from build123d import *

# Parameters (mm, degrees)
BOSS_EXTRUDE1_DEPTH     = 19.05
SKETCH2_W               = 42.164
SKETCH2_H               = 27.686
BOSS_EXTRUDE2_DEPTH     = 2.54
SKETCH3_W               = 7.0612
SKETCH3_H               = 14.986
BOSS_EXTRUDE3_DEPTH     = 6.35
CUT_EXTRUDE1_DEPTH      = 50.127067096
CUT_EXTRUDE1_DEPTH_BACK = 50.127067096
SKETCH4_R               = 1.75
FILLET2_R               = 1.27
CUT_EXTRUDE2_DEPTH      = 52.65763053
CUT_EXTRUDE2_DEPTH_BACK = 52.65763053
SKETCH5_R               = 4.7625
SKETCH6_W               = 25.4
SKETCH6_H               = 4.7625
BOSS_EXTRUDE4_DEPTH     = 9.525
FILLET3_R               = 3.175
FILLET4_R               = 1.27
FILLET6_R               = 1.27
CUT_EXTRUDE3_DEPTH      = 58.486687197
CUT_EXTRUDE3_DEPTH_BACK = 58.486687197
SKETCH8_R               = 2.3
SKETCH9_W               = 2.54
SKETCH9_H               = 10.16
CUT_EXTRUDE4_DEPTH      = 14.5288
CUT_EXTRUDE5_DEPTH      = 51.648644651
CUT_EXTRUDE5_DEPTH_BACK = 51.648644651
SKETCH10_R              = 1.7499965


with BuildPart() as part:
    # Sketch1 → Boss-Extrude1 (new body)
    with BuildSketch(Plane.XY):
        Polygon((-2.54, 25.146), (39.624, 25.146), (39.624, 22.606), (37.084, 22.606), (0, 22.606), (0, 0), (37.084, 0), (39.624, 0), (39.624, -2.54), (-2.54, -2.54), align=None)
    extrude(amount=BOSS_EXTRUDE1_DEPTH)

    # Sketch2 → Boss-Extrude2 (add)
    with BuildSketch(Plane.XY.offset(19.05)):
        with Locations((18.542, 11.303)):
            Rectangle(SKETCH2_W, SKETCH2_H)
    extrude(amount=BOSS_EXTRUDE2_DEPTH)

    # Sketch3 → Boss-Extrude3 (add)
    with BuildSketch(Plane.ZY.offset(2.54)):
        with Locations((18.0594, 11.303)):
            Rectangle(SKETCH3_W, SKETCH3_H)
    extrude(amount=BOSS_EXTRUDE3_DEPTH)

    # Sketch4 → Cut-Extrude1 (cut, two sides: drawn at the far end of the back side and taken through both)
    with BuildSketch(Plane(origin=(0, 0, 14.5288), x_dir=(-1, 0, 0), z_dir=(0, 0, -1)).offset(-CUT_EXTRUDE1_DEPTH_BACK)):
        with Locations(Location((4.7625, 11.303, 0), (0, 0, 90))):
            Circle(SKETCH4_R)
    extrude(amount=CUT_EXTRUDE1_DEPTH + CUT_EXTRUDE1_DEPTH_BACK, mode=Mode.SUBTRACT)

    # Fillet2
    fillet2_edges = [part.edges().sort_by_distance(p)[0] for p in [
        (-2.54, 18.796, 18.0594),
        (-2.54, 3.81, 18.0594),
        (-8.89, 18.796, 18.0594),
        (-8.89, 3.81, 18.0594),
    ]]
    fillet(fillet2_edges, radius=FILLET2_R)

    # Sketch5 → Cut-Extrude2 (cut, two sides: drawn at the far end of the back side and taken through both)
    with BuildSketch(Plane.XY.offset(21.59).offset(-CUT_EXTRUDE2_DEPTH_BACK)):
        with Locations((10.16, 11.303)):
            Circle(SKETCH5_R)
        with BuildLine():
            Line((25.4, 16.0655), (10.16, 16.0655))
            ThreePointArc((10.16, 16.0655), (13.527596045, 14.670596045), (14.9225, 11.303))
            ThreePointArc((14.9225, 11.303), (13.527596045, 7.935403955), (10.16, 6.5405))
            Line((10.16, 6.5405), (25.4, 6.5405))
            ThreePointArc((25.4, 6.5405), (20.6375, 11.303), (25.4, 16.0655))
        make_face()
        with Locations((25.4, 11.303)):
            Circle(SKETCH5_R)
    extrude(amount=CUT_EXTRUDE2_DEPTH + CUT_EXTRUDE2_DEPTH_BACK, mode=Mode.SUBTRACT)

    # Sketch6 → Boss-Extrude4 (add)
    with BuildSketch(Plane.XY.offset(21.59)):
        with Locations((26.924, 22.76475)):
            Rectangle(SKETCH6_W, SKETCH6_H)
    extrude(amount=BOSS_EXTRUDE4_DEPTH)

    # Fillet3
    fillet3_edges = [part.edges().sort_by_distance(p)[0] for p in [
        (14.224, 22.76475, 21.59),
        (14.224, 22.76475, 31.115),
        (39.624, 22.76475, 31.115),
    ]]
    fillet(fillet3_edges, radius=FILLET3_R)

    # Fillet4
    fillet4_edges = [part.edges().sort_by_distance(p)[0] for p in [
        (25.3365, 20.3835, 21.59),
    ]]
    fillet(fillet4_edges, radius=FILLET4_R)

    # Fillet6
    fillet6_edges = [part.edges().sort_by_distance(p)[0] for p in [
        (0, 0, 9.525),
        (0, 22.606, 9.525),
    ]]
    fillet(fillet6_edges, radius=FILLET6_R)

    # Sketch8 → Cut-Extrude3 (cut, two sides: drawn at the far end of the back side and taken through both)
    with BuildSketch(Plane(origin=(0, 25.146, 0), x_dir=(1, 0, 0), z_dir=(0, 1, 0)).offset(-CUT_EXTRUDE3_DEPTH_BACK)):
        with Locations(Location((20.574, -26.3525, 0), (0, 0, 270))):
            Circle(SKETCH8_R)
        with Locations(Location((33.274, -26.3525, 0), (0, 0, 270))):
            Circle(SKETCH8_R)
    extrude(amount=CUT_EXTRUDE3_DEPTH + CUT_EXTRUDE3_DEPTH_BACK, mode=Mode.SUBTRACT)

    # Sketch9 → Cut-Extrude4 (cut)
    with BuildSketch(Plane(origin=(0, 0, 0), x_dir=(-1, 0, 0), z_dir=(0, 0, -1))):
        with Locations((1.27, 11.303)):
            Rectangle(SKETCH9_W, SKETCH9_H)
    extrude(amount=-CUT_EXTRUDE4_DEPTH, mode=Mode.SUBTRACT)

    # Sketch10 → Cut-Extrude5 (cut, two sides: drawn at the far end of the back side and taken through both)
    with BuildSketch(Plane(origin=(0, 0, 19.05), x_dir=(-1, 0, 0), z_dir=(0, 0, -1)).offset(-CUT_EXTRUDE5_DEPTH_BACK)):
        with Locations(Location((-34.344, 1.95, 0), (0, 0, 180))):
            Circle(SKETCH10_R)
    extrude(amount=CUT_EXTRUDE5_DEPTH + CUT_EXTRUDE5_DEPTH_BACK, mode=Mode.SUBTRACT)


solid = part.part
Model file for the job. Use its own axes, mm. A direction names the side the tool comes from. Give positions to 0.01 mm unless a question says otherwise; leave off trailing zeros. Loops run counter-clockwise (first coordinate to the right, second up) from the corner with the lowest first, then second, coordinate; pieces in that order, holes last. Notation, with made-up numbers: (-35, -33) -> (-22, -33) arc R24 ccw to (-22, -9) -> close; hole circle Ø6 at (-5.75, 31). An arc over 180 degrees is marked (long way). Use a Markdown table: item, result. Add a question column.
(1) Tool access for faces 1 (the flat face through (18, 6.54, 20)), 2 (the flat face through (-1, 6.223, 7)), 3 (the cylindrical face through (0.36, 22.22, 9.66)): list every direction of +Z, -Z, +X, -X, +Y, -Y with a clear straight run to the whole face (end or side of a thin tool).
(2) Wall check: line 1 along Y through (x, z) = (17.5, 16); line 2 along Z through (x, y) = (10, 24.25); line 3 along Z through (x, y) = (33.5, 17.75). Give the ranges that are in metal, low to high.
(3) Slice it at A-A on y = 1.95. List the corners of the cut face in (x, z).
(4) Mould opens along X. For faces 4 (the flat face through (18, 16.066, 20)), 5 (the flat face through (-2.54, 21, 8)), 6 (the flat face through (27, 23, 31.115)) say: +X half, -X half, draft (parallel to the pull), parting line (faces both ways), or undercut.
(5) Drop flat-ended pins along their axis: pin 1 Ø3 at (x, y) = (14.5, 6.5) entering from +Z; pin 2 Ø2.5 at (x, z) = (25.5, 28) entering from -Y; pin 3 Ø11.5 at (x, y) = (27.5, 14) entering from -Z. Give the stop position or say it passes through.
(6) Slice it at D-D on x = -2. List the corners of the cut face in (y, z).
(7) Slice it at B-B on x = 15. List the corners of the cut face in (y, z), and give its area (3 significant figures).
(8) Slice it at C-C on z = 20. Give the number of separate pieces and of enclosed holes in the cut face, and give its area (3 significant figures).
Filled sheet:
| question | item | result |
|---|---|---|
| 1 | face 1 | +Z, -Z |
| 1 | face 2 | -Z, +X, -X |
| 1 | face 3 | -Z, +X |
| 2 | line 1 | -2.54 to 0, 22.61 to 25.15 |
| 2 | line 2 | 0 to 21.59 |
| 2 | line 3 | 19.05 to 21.59 |
| 3 | outline | (-2.54, 0) -> (0, 0) -> (0, 19.05) -> (32.59, 19.05) -> (32.59, 21.59) -> (-2.54, 21.59) -> close; (36.09, 19.05) -> (39.62, 19.05) -> (39.62, 21.59) -> (36.09, 21.59) -> close |
| 4 | face 4 | undercut |
| 4 | face 5 | -X half |
| 4 | face 6 | draft |
| 5 | pin 1 | z = 21.59 |
| 5 | pin 2 | y = 20.38 |
| 5 | pin 3 | z = 19.05 |
| 6 | outline | (-2.54, 0) -> (6.22, 0) -> (6.22, 14.53) -> (16.38, 14.53) -> (16.38, 0) -> (25.15, 0) -> (25.15, 21.59) -> (-2.54, 21.59) -> close |
| 7 | outline | (-2.54, 0) -> (0, 0) -> (0, 19.05) -> (6.54, 19.05) -> (6.54, 21.59) -> (-2.54, 21.59) -> close; (16.07, 19.05) -> (22.61, 19.05) -> (22.61, 0) -> (25.15, 0) -> (25.15, 30.02) -> (20.38, 30.02) -> (20.38, 22.86) arc R1.27 cw to (19.11, 21.59) -> (16.07, 21.59) -> close |
| 7 | area | 183 mm2 |
| 8 | separate pieces | 1 |
| 8 | enclosed holes | 3 |
| 8 | area | 1,030 mm2 |
